Check sheet for the modelled part. Datum: model origin and axes. Units: mm. A direction names the side the tool comes from. Coordinates: 2 decimals unless noted, no trailing zeros. Loops run counter-clockwise (first coordinate to the right, second up) from the corner with the lowest first, then second, coordinate; pieces in that order, holes last.
from build123d import *

# Parameters (mm, degrees)
SKETCH1_W           = 33
SKETCH1_H           = 50
BOSS_EXTRUDE1_DEPTH = 8
SKETCH2_W           = 12
SKETCH2_H           = 10
BOSS_EXTRUDE2_DEPTH = 12
FILLET1_R           = 4
FILLET2_R           = 4
SKETCH3_R           = 2.75
SKETCH3_R_2         = 11.6
CUT_EXTRUDE1_DEPTH  = 104.266645155
BOSS_EXTRUDE3_START = 0.5
SKETCH4_R           = 4.25
SKETCH4_R_2         = 2.75
BOSS_EXTRUDE3_DEPTH = 0.5
SKETCH7_R           = 2.75
CUT_EXTRUDE3_DEPTH  = 104.653268207
SKETCH6_R           = 12.1
CUT_EXTRUDE2_DEPTH  = 5.1
CHAMFER1_SIZE       = 2.5


with BuildPart() as part:
    # Sketch1 → Boss-Extrude1 (new body)
    with BuildSketch(Plane.XY):
        with Locations((61.5, 25)):
            Rectangle(SKETCH1_W, SKETCH1_H)
    extrude(amount=BOSS_EXTRUDE1_DEPTH)

    # Sketch2 → Boss-Extrude2 (add)
    with BuildSketch(Plane(origin=(0, 0, 0), x_dir=(-1, 0, 0), z_dir=(0, 0, -1))):
        with Locations((-84, 45)):
            Rectangle(SKETCH2_W, SKETCH2_H)
        with Locations((-84, 5)):
            Rectangle(SKETCH2_W, SKETCH2_H)
    extrude(amount=-BOSS_EXTRUDE2_DEPTH)

    # Fillet1
    fillet1_edges = [part.edges().sort_by_distance(p)[0] for p in [
        (78, 40, 4),
        (78, 10, 4),
    ]]
    fillet(fillet1_edges, radius=FILLET1_R)

    # Fillet2
    fillet2_edges = [part.edges().sort_by_distance(p)[0] for p in [
        (78, 5, 8),
        (80, 10, 8),
        (78, 45, 8),
        (80, 40, 8),
    ]]
    fillet(fillet2_edges, radius=FILLET2_R - 0.0001)  # a hair under: the kernel refuses the full size

    # Sketch3 → Cut-Extrude1 (cut, through all)
    with BuildSketch(Plane.XY.offset(8)):
        with Locations((69.99999756, 15.000000247)):
            Circle(SKETCH3_R)
        with Locations((45, 35)):
            Circle(SKETCH3_R_2)
        with BuildLine():
            Line((27.5, 35), (12.5, 35))
            ThreePointArc((12.5, 35), (26.943967427, 7.9772376), (57.437211552, 4.973915193))
            ThreePointArc((57.437211552, 4.973915193), (61.496182303, 14.77313743), (51.696960066, 18.832108181))
            ThreePointArc((51.696960066, 18.832108181), (35.277520922, 20.449281785), (27.5, 35))
        make_face()
    extrude(amount=-CUT_EXTRUDE1_DEPTH, mode=Mode.SUBTRACT)

    # Sketch4 → Boss-Extrude3 (add)
    with BuildSketch(Plane.XY.offset(8).offset(BOSS_EXTRUDE3_START)):
        with Locations(Location((69.99999756, 15.000000247, 0), (0, 0, 340.25017454))):
            Circle(SKETCH4_R)
        with Locations((69.99999756, 15.000000247)):
            Circle(SKETCH4_R_2, mode=Mode.SUBTRACT)
    extrude(amount=-BOSS_EXTRUDE3_DEPTH)

    # Sketch7 → Cut-Extrude3 (cut, through all)
    with BuildSketch(Plane(origin=(0, 50, 0), x_dir=(1, 0, 0), z_dir=(0, 1, 0))):
        with Locations(Location((84, -6, 0), (0, 0, 180))):
            Circle(SKETCH7_R)
    extrude(amount=-CUT_EXTRUDE3_DEPTH, mode=Mode.SUBTRACT)

    # Mirror1: part across plane


with BuildPart() as part_1:
    add(part.part)
    add(part.part.mirror(Plane(origin=(45, 50, 8), x_dir=(0, 0, 1), z_dir=(1, 0, 0))))

    # Sketch6 → Cut-Extrude2 (cut)
    with BuildSketch(Plane(origin=(0, 0, 0), x_dir=(-1, 0, 0), z_dir=(0, 0, -1))):
        with Locations((-45, 35)):
            Circle(SKETCH6_R)
    extrude(amount=-CUT_EXTRUDE2_DEPTH, mode=Mode.SUBTRACT)

    # Chamfer1
    chamfer1_edges = [part_1.edges().sort_by_distance(p)[0] for p in [
        (22.75000244, 15.000000247, 0),
        (67.24999756, 15.000000247, 0),
    ]]
    chamfer(chamfer1_edges, length=CHAMFER1_SIZE)


solid = part_1.part
(1) Section check B-B, the plane x = 6. Enter the section's corners in (y, z), plus the area to 3 significant figures.
(2) Gauge pin test, flat ends, axial feed: P1, Ø5, axis at x = 20, y = 9, coming from the -Z side; P2, Ø4, axis at y = 29.5, z = 5, coming from the +X side; P3, Ø6, axis at y = 36, z = 6, coming from the -X side; P4, Ø6, axis at x = 54, y = 20, coming from the +Z side. Record the tip position at first contact, or that the pin passes through.
(3) Section check C-C, the plane y = 8.5. Count the separate pieces of the cut face and the enclosed holes in it, plus the area to 3 significant figures.
(4) Scan lines: line 1 along Y through (x, z) = (44.5, 1.5); line 2 along Y through (x, z) = (45, 6.45); line 3 along X through (y, z) = (35, 6.65). Record each from-to range of solid material in increasing order.
(5) Section check D-D, the plane z = 1.5. Enter the section's corners in (x, y).
(6) Set-up check for faces 1 (the face through (10.859, 38.797, 4.751)), 2 (the face through (38, 25, 8)), 3 (the face through (87, 10, 6)), 4 (the face through (21, 12, 8.5)): record each of +Z, -Z, +X, -X, +Y, -Y from which the full face is reachable in a straight line by a thin tool's end or side.
(7) Section check A-A, the plane y = 35. Enter the section's corners in (x, z), plus the area to 3 significant figures.
(8) Draft check along X on faces 5 (the face through (87, 40, 6)), 6 (the face through (86.747, 5.106, 6.121)), 7 (the face through (79.141, 11.203, 4.751)). Enter one of: pulls with the +X half, pulls with the -X half, needs draft (parallel to the pull), parting line crosses it, or undercut.
Determined:
1. outline: (0, 0) - (10, 0) - (10, 3.25) - (0, 3.25) - close; (0, 8.75) - (10, 8.75) - (10, 12) - (0, 12) - close; (40, 0) - (50, 0) - (50, 3.25) - (40, 3.25) - close; (40, 8.75) - (50, 8.75) - (50, 12) - (40, 12) - close
1. area: 130 mm2
2. P1: stops at z = 0
2. P2: stops at x = 78
2. P3: stops at x = 10.65
2. P4: stops at z = 8
3. separate pieces: 2
3. enclosed holes: 2
3. area: 515 mm2
4. line 1: y = 0 to 2.5, 17.51 to 22.91, 47.09 to 50
4. line 2: y = 0 to 2.5, 17.5 to 23.4, 46.6 to 50
4. line 3: x = 12 to 33.4, 56.6 to 78
5. outline: (0, 0) - (90, 0) - (90, 10) - (82, 10) arc R4 cw to (78, 14) - (78, 36) arc R4 cw to (82, 40) - (90, 40) - (90, 50) - (0, 50) - (0, 40) - (8, 40) arc R4 cw to (12, 36) - (12, 14) arc R4 cw to (8, 10) - (0, 10) - close; hole circle Ø7.5 at (20, 15); hole (32.56, 4.97) arc R32.5 ccw to (57.44, 4.97) arc R7.5 ccw to (51.7, 18.83) arc R17.5 cw to (38.3, 18.83) arc R7.5 ccw to start; hole circle Ø24.2 at (45, 35); hole circle Ø7.5 at (70, 15)
6. face 1: +Z, -Z, -X
6. face 2: +Z
6. face 3: +Z, -Z, +X
6. face 4: +Z, +Y, -Y
7. outline: (12, 0) - (32.9, 0) - (32.9, 5.1) - (33.4, 5.1) - (33.4, 8) - (12, 8) - close; (56.6, 5.1) - (57.1, 5.1) - (57.1, 0) - (78, 0) - (78, 8) - (56.6, 8) - close
7. area: 337 mm2
8. face 5: needs draft
8. face 6: undercut
8. face 7: pulls with the +X half
